```python
from build123d import *

# Parameters (mm, degrees)
SKETCH3_R           = 1
BOSS_EXTRUDE2_DEPTH = 5


with BuildPart() as part:
    # Sketch3 → Boss-Extrude2 (new body)
    with BuildSketch(Plane(origin=(0, 0, 0), x_dir=(1, 0, 0), z_dir=(0, 1, 0))):
        with BuildLine():
            Line((-5, 40), (-5, 0))
            ThreePointArc((-5, 0), (-4.619397663, -1.913417162), (-3.535533906, -3.535533906))
            Line((-3.535533906, -3.535533906), (17.67766953, -24.748737342))
            ThreePointArc((17.67766953, -24.748737342), (24.748737342, -24.748737342), (24.748737342, -17.67766953))
            Line((24.748737342, -17.67766953), (5, 2.071067812))
            Line((5, 2.071067812), (5, 40))
            ThreePointArc((5, 40), (0, 45), (-5, 40))
        make_face()
        with Locations(Location((0, 0, 0), (0, 0, 270))):
            Circle(SKETCH3_R, mode=Mode.SUBTRACT)
        with Locations(Location((21.213203436, -21.213203436, 0), (0, 0, 270))):
            Circle(SKETCH3_R, mode=Mode.SUBTRACT)
    extrude(amount=BOSS_EXTRUDE2_DEPTH)


solid = part.part
```
Can you work these out from the model? Positions are in its coordinate system, mm. Round coordinates to 2 decimals unless told otherwise and drop trailing zeros. Loops run counter-clockwise (first coordinate to the right, second up) from the corner with the lowest first, then second, coordinate; pieces in that order, holes last. Notation, with made-up numbers: M 4,32 L 50,32 A21 ccw 50,71 Z; hole C 40,15.25 d7. An arc over 180 degrees is marked long. Answer in a Markdown table with one row per item.
1. If we section it at C-C, the plane z = -26: Please give me the cut outline in (x, y).
Established:
| item | result |
|---|---|
| outline | M -5,0 L 5,0 L 5,5 L -5,5 Z |
2. Please list where these lines run through material, in increasing order: line 1 (X direction, y = 4.25, z = -21); line 2 (X direction, y = 1.85, z = 0); line 3 (X direction, y = 4.45, z = 9). Write a range as from..to.
Established:
| item | result |
|---|---|
| line 1 | -5..5 |
| line 2 | -5..-1, 1..7.07 |
| line 3 | 1.93..16.07 |
3. If we section it at B-B, the plane y = 2.3: Please give me the cut outline in (x, z).
Established:
| item | result |
|---|---|
| outline | M -5,-40 A5 ccw 5,-40 L 5,-2.07 L 24.75,17.68 A5 ccw 17.68,24.75 L -3.54,3.54 A5 ccw -5,0 Z; hole C 0,0 d2; hole C 21.21,21.21 d2 |
4. If we section it at D-D, the plane x = 8: Please give me the cut outline in (y, z), plus the area to 3 significant figures.
Established:
| item | result |
|---|---|
| outline | M 0,0.93 L 5,0.93 L 5,15.07 L 0,15.07 Z |
| area | 70.7 mm² |
5. Thinking about a two-plate mould opening in X: for faces 1 (the face through (5, 2, -21)), 2 (the face through (0, 2, -45)), 3 (the face through (-1, 2, 0)), which applies, pulls with the +X half, pulls with the -X half, needs draft (parallel to the pull), parting line crosses it, or undercut?
Established:
| item | result |
|---|---|
| face 1 | pulls with the +X half |
| face 2 | parting line crosses it |
| face 3 | undercut |
6. If we section it at A-A, the plane x = 0: Please give me the cut outline in (y, z).
Established:
| item | result |
|---|---|
| outline | M 0,-45 L 5,-45 L 5,-1 L 0,-1 Z; M 0,1 L 5,1 L 5,7.07 L 0,7.07 Z |
7. I'm going to push flat-ended pins straight in: pin 1 Ø3 at (y, z) = (3, 18) entering from -X; pin 2 Ø2 at (x, y) = (4.5, 3.5) entering from -Z; pin 3 Ø1.5 at (y, z) = (3.5, -26.5) entering from +X. Where does each tip first touch, or does it pass through?
Established:
| item | result |
|---|---|
| pin 1 | x = 9.43 |
| pin 2 | z = -43.57 |
| pin 3 | x = 5 |
